from build123d import *

# Parameters (mm, degrees)
PAD_DEPTH = 100


with BuildPart() as part:
    # Sketch → Pad (new body)
    with BuildSketch(Plane.YZ):
        Polygon((0, 0), (20, 0), (20, 3), (3, 3), (3, 20), (0, 20), align=None)
    extrude(amount=PAD_DEPTH)


solid = part.part
Work out the finished part from the listing and answer in its coordinate system (mm). A direction names the side the tool comes from. Round coordinates to 2 decimals unless told otherwise and drop trailing zeros. Order: outer loops, then holes, each group sorted by start corner. A loop starts at its lowest first (then second) coordinate and runs counter-clockwise, first axis right, second up. Notation, with made-up numbers: M 69,77.25 L 118,77.25 A32 ccw 118,104.25 Z; hole C 64.5,23.25 d1. An arc over 180 degrees is marked long. Put each result on its own line as item: value. Start each with the question number.
Q1. Flat-ended cylindrical pins translate along their axes: pin 1 (8.5 mm diameter, centred on x = 49.5, y = 7.5, fed in from +Z); pin 2 (5 mm diameter, centred on x = 65, z = 14.5, fed in from +Y). Find the tip coordinate at first contact, or state that the pin passes through.
Q2. A straight line is drawn through the part: L1, parallel to Z at x = 15.5, y = 4.25. Find the intervals that lie inside material, in ascending order. Write a range as [from, to].
Q3. A tool of negligible diameter and unlimited length cuts with its end or side. For faces 1 (the flat face through (49, 20, 1)), 2 (the flat face through (49, 3, 11)), from which of +Z, -Z, +X, -X, +Y, -Y can it reach the whole face along a straight path? Write none if from no direction.
Q4. Section B-B, the plane y = 4.5 is taken. Write down the section's boundary in (x, z), and give its area (3 significant figures).
Q5. Section A-A, the plane x = 46.5 is taken. Write down the section's boundary in (y, z).
Findings below:
1. pin 1: stops at z = 3
1. pin 2: stops at y = 3
2. L1: z = [0, 3]
3. face 1: +Z, -Z, +X, -X, +Y
3. face 2: +Z, +X, -X, +Y
4. outline: M 0,0 L 100,0 L 100,3 L 0,3 Z
4. area: 300 mm^2
5. outline: M 0,0 L 20,0 L 20,3 L 3,3 L 3,20 L 0,20 Z
